from build123d import *

# Parameters (mm, degrees)
SKETCH_R  = 6
PAD_DEPTH = 7.5
FILLET_R  = 1.5


with BuildPart() as part:
    # Sketch → Pad (new body)
    with BuildSketch(Plane.YZ):
        Circle(SKETCH_R)
        with BuildLine():
            ThreePointArc((-0.75, 4.234088), (0, 3.895526), (0.75, 4.234088))
            ThreePointArc((4.234088, 0.75), (3.040559, 3.040559), (0.75, 4.234088))
            ThreePointArc((4.234088, 0.75), (3.895526, 0), (4.234088, -0.75))
            ThreePointArc((0.75, -4.234088), (3.040559, -3.040559), (4.234088, -0.75))
            ThreePointArc((0.75, -4.234088), (0, -3.895526), (-0.75, -4.234088))
            ThreePointArc((-4.234088, -0.75), (-3.040559, -3.040559), (-0.75, -4.234088))
            ThreePointArc((-4.234088, -0.75), (-3.895526, 0), (-4.234088, 0.75))
            ThreePointArc((-0.75, 4.234088), (-3.040559, 3.040559), (-4.234088, 0.75))
        make_face(mode=Mode.SUBTRACT)
    extrude(amount=PAD_DEPTH)

    # Fillet
    fillet_edges = [part.edges().sort_by_distance(p)[0] for p in [
        (7.5, -6, 0),
    ]]
    fillet(fillet_edges, radius=FILLET_R)


solid = part.part
Part model, mm, in its own coordinate system. Coordinates: 2 decimals unless noted, no trailing zeros. Loops run counter-clockwise (first coordinate to the right, second up) from the corner with the lowest first, then second, coordinate; pieces in that order, holes last. Notation, with made-up numbers: M -28.5,17 L -9.5,17 A37 ccw -9.5,56 Z; hole C 76,14 d6. An arc over 180 degrees is marked long. Use a Markdown table: item, result. Add a question column.
Q1. Cut at A-A (x = 1). Write the cut outline in (y, z).
Q2. Probe L1, parallel to Y at x = 2, z = -3.5; L2, parallel to Y at x = 7, z = 3.25; L3, parallel to Z at x = 7, y = 1.5. List the from-to ranges inside material, lowest first.
Q3. Cut at B-B (z = 0). Write the cut outline in (x, y), and give its area (3 significant figures).
Q4. Pin check, flat tips, straight feed: P1, Ø1, axis at x = 6.5, z = -3, coming from the +Y side; P2, Ø4, axis at x = 2, z = 4, coming from the -Y side. Stop position of each tip, or through.
Q5. Mould opens along Y. For faces 1 (the cylindrical face through (3.698, -3.896, -0.012)), 2 (the cylindrical face through (3, -6, 0)), 3 (the flat face through (0, -4.1, 0.1)) say: +Y half, -Y half, draft (parallel to the pull), parting line (faces both ways), or undercut.
Worked out:
| question | item | result |
|---|---|---|
| 1 | outline | C 0,0 d12; hole M -4.23,-0.75 A4.3 ccw -0.75,-4.23 A1 cw 0.75,-4.23 A4.3 ccw 4.23,-0.75 A1 cw 4.23,0.75 A4.3 ccw 0.75,4.23 A1 cw -0.75,4.23 A4.3 ccw -4.23,0.75 A1 cw Z |
| 2 | L1 | y = -4.87 to -2.5, 2.5 to 4.87 |
| 2 | L2 | y = -4.58 to -2.82, 2.82 to 4.58 |
| 2 | L3 | z = -5.41 to -4.03, 4.03 to 5.41 |
| 3 | outline | M 0,-6 L 6,-6 A1.5 ccw 7.5,-4.5 L 7.5,-3.9 L 0,-3.9 Z; M 0,3.9 L 7.5,3.9 L 7.5,4.5 A1.5 ccw 6,6 L 0,6 Z |
| 3 | area | 30.6 mm2 |
| 4 | P1 | stops at y = 5.4 |
| 4 | P2 | stops at y = -5.66 |
| 5 | face 1 | undercut |
| 5 | face 2 | parting line |
| 5 | face 3 | draft |
